Here's how the part is built. I have some questions about the finished solid (model axes, mm). A direction names the side the tool comes from. Round coordinates to 2 decimals unless told otherwise and drop trailing zeros. Order: outer loops, then holes, each group sorted by start corner. A loop starts at its lowest first (then second) coordinate and runs counter-clockwise, first axis right, second up. Notation, with made-up numbers: M 38.5,17.25 L 80.5,17.25 A27 ccw 80.5,48.25 Z; hole C -21.5,84 d8. An arc over 180 degrees is marked long. Use one line per item in the form item = value. Start each with the question number.
```python
from build123d import *

# Parameters (mm, degrees)
SKETCH1_R                = 11.125
BOSS_EXTRUDE2_DEPTH      = 8
SKETCH2_R                = 10
BOSS_EXTRUDE3_DEPTH      = 2
BOSS_EXTRUDE6_DEPTH      = 8.66
BOSS_EXTRUDE6_DEPTH_BACK = 8.660254
CUT_EXTRUDE2_DEPTH       = 62.226087838
CUT_EXTRUDE2_DEPTH_BACK  = 62.226087838
SKETCH8_R                = 1.5
SKETCH9_W                = 30.003485383
SKETCH9_H                = 17.320254038
BOSS_EXTRUDE7_DEPTH      = 5


with BuildPart() as part:
    # Sketch1 → Boss-Extrude2 (new body)
    with BuildSketch(Plane.XY):
        Polygon((0, 17.320508076), (-15, 8.660254038), (-15, -8.660254038), (0, -17.320508076), (15, -8.660254038), (15, 8.660254038), align=None)
        Circle(SKETCH1_R, mode=Mode.SUBTRACT)
    extrude(amount=BOSS_EXTRUDE2_DEPTH)

    # Sketch2 → Boss-Extrude3 (add)
    with BuildSketch(Plane.XY.offset(8)):
        Polygon((0, 17.320508076), (-15, 8.660254038), (-15, -8.660254038), (0, -17.320508076), (15, -8.660254038), (15, 8.660254038), align=None)
        Circle(SKETCH2_R, mode=Mode.SUBTRACT)
    extrude(amount=BOSS_EXTRUDE3_DEPTH)

    # Sketch6 → Boss-Extrude6 (add, two sides: drawn at the far end of the back side and taken through both)
    with BuildSketch(Plane(origin=(0, 0, 0), x_dir=(1, 0, 0), z_dir=(0, 1, 0)).offset(-BOSS_EXTRUDE6_DEPTH_BACK)):
        Polygon((15, -10), (15, -27.6), (20.034456679, -41.432056045), (15.330091147, -43.144305069), (10, -28.5), (10, -10), align=None)
        Polygon((-15, -10), (-15, -32.9), (-8.159597133, -51.693852416), (-3.455231601, -49.981603391), (-10, -32), (-10, -10), align=None)
    extrude(amount=BOSS_EXTRUDE6_DEPTH + BOSS_EXTRUDE6_DEPTH_BACK)

    # Sketch8 → Cut-Extrude2 (cut, two sides: drawn at the far end of the back side and taken through both)
    with BuildSketch(Plane.XZ.offset(8.660254038).offset(-CUT_EXTRUDE2_DEPTH_BACK)):
        with Locations(Location((-10.44787914, 38.088155725, 0), (0, 0, 90))):
            Circle(SKETCH8_R)
        with Locations(Location((-7.175494941, 47.07895742, 0), (0, 0, 90))):
            Circle(SKETCH8_R)
        with Locations(Location((16.31419334, 38.529410074, 0), (0, 0, 270))):
            Circle(SKETCH8_R)
        with Locations(Location((13.868080573, 31.808770483, 0), (0, 0, 270))):
            Circle(SKETCH8_R)
    extrude(amount=CUT_EXTRUDE2_DEPTH + CUT_EXTRUDE2_DEPTH_BACK, mode=Mode.SUBTRACT)

    # Sketch9 → Boss-Extrude7 (add)
    with BuildSketch(Plane(origin=(15.659592369, 0, 43.024376432), x_dir=(0.9396926207859078, 0, -0.3420201433256706), z_dir=(0.3420201433256706, 0, 0.9396926207859078))):
        with Locations((-10.346109336, -0.000127019)):
            Rectangle(SKETCH9_W, SKETCH9_H)
    extrude(amount=BOSS_EXTRUDE7_DEPTH)


solid = part.part
```
1) If I drill on line 1 (X direction, y = -8, z = 20); line 2 (X direction, y = -0.5, z = 31); line 3 (Y direction, x = 10.5, z = 46), over which ranges is the centre line in solid material (lowest first)?
2) If we section it at A-A on z = 22.5: Write out the boundary of the cut face in (x, y), then the cut area to 3 significant figures.
3) If we mould it in two halves opening along Z, with no side actions, what happens to faces 4 (the flat face through (12, 8.66, 32)), 5 (the flat face through (7.45, 0.121, 51.333)), 6 (the flat face through (-10, 2, 8)), 7 (the flat face through (0, -11, 10))? For each: +Z half, -Z half, draft (parallel to the pull), parting line (faces both ways), or undercut.
4) Will these pins go through, and if not, where does the flat tip stop? pin 1 Ø13.5 at (x, y) = (0, 0) entering from +Z; pin 2 Ø6 at (x, y) = (-8, -0.5) entering from -Z; pin 3 Ø4 at (x, z) = (-7.18, 47.08) entering from -Y.
5) If we section it at C-C on y = 7.5: Write out the boundary of the cut face in (x, z), then the cut area to 3 significant figures.
6) If we section it at B-B on x = 5: Write out the boundary of the cut face in (y, z).
7) If we section it at D-D on y = -14: Write out the boundary of the cut face in (x, z), then the cut area to 3 significant figures.
8) On a 3-axis mill with a long thin cutter (end or side, diameter ignored), from which of +Z, -Z, +X, -X, +Y, -Y can I reach the whole of each face in a straight line? I mean faces 1 (the flat face through (-10, 0, 21)), 2 (the cylindrical face through (-8.2, 7.52, 3.94)), 3 (the flat face through (12, -8.66, 32)). Say none if no direction works.
Completed:
q1.line_1 = -15 to -10, 10 to 15
q1.line_2 = -15 to -10, 10.91 to 12.6, 15.13 to 16.24
q1.line_3 = -8.66 to 8.66
q2.outline = M -15,-8.66 L -10,-8.66 L -10,8.66 L -15,8.66 Z; M 10,-8.66 L 15,-8.66 L 15,8.66 L 10,8.66 Z
q2.area = 173 mm²
q3.face_4 = draft
q3.face_5 = +Z half
q3.face_6 = -Z half
q3.face_7 = undercut
q4.pin_1 = 56.39
q4.pin_2 = 8
q4.pin_3 = -8.66
q5.outline = M -15,0 L -8.22,0 L -8.22,8 L -6.61,8 L -6.61,10 L -10,10 L -10,32 L -3.46,49.98 L 15.33,43.14 L 10,28.5 L 10,10 L 6.61,10 L 6.61,8 L 8.22,8 L 8.22,0 L 15,0 L 15,27.6 L 21.74,46.13 L -6.45,56.39 L -15,32.9 Z; hole C -10.45,38.09 d3; hole C -7.18,47.08 d3; hole C 13.87,31.81 d3; hole C 16.31,38.53 d3
q5.area = 640 mm²
q6.outline = M -14.43,0 L -9.94,0 L -9.94,8 L -8.66,8 L -8.66,10 L -14.43,10 Z; M -8.66,46.9 L 8.66,46.9 L 8.66,52.23 L -8.66,52.23 Z; M 8.66,8 L 9.94,8 L 9.94,0 L 14.43,0 L 14.43,10 L 8.66,10 Z
q7.outline = M -5.75,0 L 5.75,0 L 5.75,10 L -5.75,10 Z
q7.area = 115 mm²
q8.face_1 = +Y, -Y
q8.face_2 = -Z
q8.face_3 = +Z, +X, -X, -Y
